```python
from build123d import *

# Parameters (mm, degrees)
BOSS_EXTRUDE1_DEPTH     = 152.4
CUT_EXTRUDE1_START      = -6.35
CUT_EXTRUDE1_DEPTH      = 6.35
CUT_EXTRUDE2_DEPTH      = 154.454683865
CUT_EXTRUDE2_DEPTH_BACK = 154.454683865
SKETCH4_W               = 35.4
SKETCH4_H               = 35.921024484
SKETCH5_W               = 49.45
SKETCH5_H               = 25.4
CUT_EXTRUDE3_DEPTH      = 156.02325632


with BuildPart() as part:
    # Sketch2 → Boss-Extrude1 (new, symmetric)
    with BuildSketch(Plane.XY):
        with BuildLine():
            Line((-12.7, -12.7), (12.7, -12.7))
            Line((12.7, -12.7), (12.7, 12.7))
            Line((12.7, 12.7), (11.0749969, 12.7))
            ThreePointArc((11.0749969, 12.7), (9.925946189, 12.224047611), (9.4499938, 11.0749969))
            Line((9.4499938, 11.0749969), (9.4499938, -6.2749938))
            ThreePointArc((9.4499938, -6.2749938), (8.52005783, -8.52005783), (6.2749938, -9.4499938))
            Line((6.2749938, -9.4499938), (-11.0749969, -9.4499938))
            ThreePointArc((-11.0749969, -9.4499938), (-12.224047611, -9.925946189), (-12.7, -11.0749969))
            Line((-12.7, -11.0749969), (-12.7, -12.7))
        make_face()
    extrude(amount=BOSS_EXTRUDE1_DEPTH, both=True)

    # Sketch3 → Cut-Extrude1 (cut)
    with BuildSketch(Plane(origin=(0, 0, -152.4), x_dir=(-1, 0, 0), z_dir=(0, 0, -1)).offset(CUT_EXTRUDE1_START)):
        with BuildLine():
            Line((12.7, -12.7), (12.7, -11.0749969))
            ThreePointArc((12.7, -11.0749969), (12.224047611, -9.925946189), (11.0749969, -9.4499938))
            Line((11.0749969, -9.4499938), (-6.2749938, -9.4499938))
            ThreePointArc((-6.2749938, -9.4499938), (-8.52005783, -8.52005783), (-9.4499938, -6.2749938))
            Line((-9.4499938, -6.2749938), (-9.4499938, 11.0749969))
            ThreePointArc((-9.4499938, 11.0749969), (-9.925946189, 12.224047611), (-11.0749969, 12.7))
            Line((-11.0749969, 12.7), (-12.7, 12.7))
            Line((-12.7, 12.7), (-12.7, -12.7))
            Line((-12.7, -12.7), (12.7, -12.7))
        make_face()
    extrude(amount=CUT_EXTRUDE1_DEPTH, mode=Mode.SUBTRACT)

    # Sketch4 → Cut-Extrude2 (cut, two sides: drawn at the far end of the back side and taken through both)
    with BuildSketch(Plane(origin=(0, 0, 0), x_dir=(0, 0, -1), z_dir=(0.7071067811865476, -0.7071067811865475, 0)).offset(-CUT_EXTRUDE2_DEPTH_BACK)):
        with Locations((128.35, 0)):
            Rectangle(SKETCH4_W, SKETCH4_H)
    extrude(amount=CUT_EXTRUDE2_DEPTH + CUT_EXTRUDE2_DEPTH_BACK, mode=Mode.SUBTRACT)

    # Sketch5 → Cut-Extrude3 (cut, through all)
    with BuildSketch(Plane(origin=(12.7, 0, 0), x_dir=(0, 0, -1), z_dir=(1, 0, 0))):
        with Locations((-127.675, 0)):
            Rectangle(SKETCH5_W, SKETCH5_H)
    extrude(amount=-CUT_EXTRUDE3_DEPTH, mode=Mode.SUBTRACT)


solid = part.part
```
Check sheet for the modelled part. Datum: model origin and axes. Units: mm. A direction names the side the tool comes from. Round coordinates to 2 decimals unless told otherwise and drop trailing zeros. Loops run counter-clockwise (first coordinate to the right, second up) from the corner with the lowest first, then second, coordinate; pieces in that order, holes last. Notation, with made-up numbers: M 22.5,-21.75 L 64.5,-21.75 A9 cw 64.5,-17.75 Z; hole C 28.25,-5 d3. An arc over 180 degrees is marked long. Answer as a JSON object with one key per item and string values.
1. Section check C-C (x = 1.75). Record the boundary of the cut face in (y, z).
Reply:
{"outline": "M -12.7,-110.65 L -9.45,-110.65 L -9.45,102.95 L -12.7,102.95 Z"}
2. Scan lines: line 1 (Y direction, x = -4.5, z = -95); line 2 (X direction, y = -2.5, z = -94.5); line 3 (X direction, y = 11.25, z = -84). Record each from-to range of solid material in increasing order.
Reply:
{"line 1": "y = -12.7 to -9.45", "line 2": "x = 9.45 to 12.7", "line 3": "x = 9.46 to 12.7"}
3. Section check B-B (y = 7.75). Record the boundary of the cut face in (x, z), plus the area to 3 significant figures.
Reply:
{"outline": "M 9.45,-110.65 L 12.7,-110.65 L 12.7,102.95 L 9.45,102.95 Z", "area": "694 mm²"}
4. Gauge pin test, flat ends, axial feed: P1, Ø5, axis at y = 0.5, z = -43.5, coming from the -X side; P2, Ø6, axis at x = 4.5, z = 21, coming from the +Y side; P3, Ø1.5, axis at y = -6.5, z = -83, coming from the -X side; P4, Ø5, axis at x = -2.5, y = -4.5, coming from the +Z side. Record the tip position at first contact, or that the pin passes through.
Reply:
{"P1": "stops at x = 9.45", "P2": "stops at y = -9.2", "P3": "stops at x = 9.3", "P4": "passes through"}
5. Access from +Z, -Z, +X, -X, +Y, -Y to the whole of each face (thin tool, end or side, straight path). Record for faces 1 (the flat face through (-2, -9.45, -2)), 2 (the flat face through (6, -10, 102.95)).
Reply:
{"face 1": "+Z, -Z, -X, +Y", "face 2": "+Z, +X, -X, +Y, -Y"}
6. Section check A-A (z = -58.5). Record the boundary of the cut face in (x, y) (3 decimals), plus the area to 3 significant figures.
Reply:
{"outline": "M -12.7,-12.7 L 12.7,-12.7 L 12.7,12.7 L 11.075,12.7 A1.625 ccw 9.45,11.075 L 9.45,-6.275 A3.175 cw 6.275,-9.45 L -11.075,-9.45 A1.625 ccw -12.7,-11.075 Z", "area": "156 mm²"}
